Design review of the part built by this model. Coordinates are the model's own, in mm. Round coordinates to 2 decimals unless told otherwise and drop trailing zeros. Order: outer loops, then holes, each group sorted by start corner. A loop starts at its lowest first (then second) coordinate and runs counter-clockwise, first axis right, second up. Notation, with made-up numbers: (-11, -23) - (33, -23) arc R33 cw to (33, 5) - close; hole circle Ø4 at (-25.5, 47.5). An arc over 180 degrees is marked (long way). Use CSV: the item, a comma, the result in double quotes.
from build123d import *

# Parameters (mm, degrees)
SKETCH_1_W                = 188
SKETCH_1_H                = 150
EXTRUDE_1_DEPTH           = 2
SKETCH_13_W               = 188
SKETCH_13_H               = 12
CUT_EXTRUDE_8_DEPTH       = 11
SKETCH_5_R                = 1
EPP_DEPTH                 = 2
SKETCH_6_R                = 1
CUT_EXTRUDE_4_DEPTH       = 2
B_FAN_DEPTH               = 2
PCI_E_DEPTH               = 2
SKETCH_14_R               = 1
CUT_EXTRUDE_7447_DEPTH    = 5
IO_2_DEPTH                = 10
HOLE_WIZARD_1_AT_2_COUNT  = 2
HOLE_WIZARD_1_AT_2_PITCH  = 115.8
HOLE_WIZARD_1_AT_3_COUNT  = 2
HOLE_WIZARD_1_AT_3_PITCH  = 132.697701563
HOLE_WIZARD_1_AT_4_COUNT  = 2
HOLE_WIZARD_1_AT_4_PITCH  = 105.840068027
HOLE_WIZARD_1_AT_5_COUNT  = 2
HOLE_WIZARD_1_AT_5_PITCH  = 150.067318228
HOLE_WIZARD_1_AT_6_COUNT  = 2
HOLE_WIZARD_1_AT_6_PITCH  = 108.209056922
HOLE_WIZARD_1_AT_7_COUNT  = 2
HOLE_WIZARD_1_AT_7_PITCH  = 19.776754031
HOLE_WIZARD_1_AT_8_COUNT  = 2
HOLE_WIZARD_1_AT_8_PITCH  = 114.604799201
HOLE_WIZARD_1_AT_9_COUNT  = 2
HOLE_WIZARD_1_AT_9_PITCH  = 163.276483304
HOLE_WIZARD_1_AT_10_COUNT = 2
HOLE_WIZARD_1_AT_10_PITCH = 128.548084389
CUT_EXTRUDE_14_DEPTH      = 10
FILLET_2_R                = 1


with BuildPart() as part:
    # 草图1 → 凸台-拉伸1 (new body)
    with BuildSketch(Plane(origin=(0, 0, 0), x_dir=(0, 0, -1), z_dir=(1, 0, 0))):
        with Locations((-63.845257573, 68.271545487)):
            Rectangle(SKETCH_1_W, SKETCH_1_H)
    extrude(amount=EXTRUDE_1_DEPTH)

    # 草图13 → 切除-拉伸8 (cut)
    with BuildSketch(Plane(origin=(2, 0, 0), x_dir=(0, 0, -1), z_dir=(1, 0, 0))):
        with Locations((-63.845257573, 137.271545487)):
            Rectangle(SKETCH_13_W, SKETCH_13_H)
    extrude(amount=-CUT_EXTRUDE_8_DEPTH, mode=Mode.SUBTRACT)

    # 草图5 → EPP (cut)
    with BuildSketch(Plane.ZY):
        with Locations((40.345257573, 125.671545487)):
            Circle(SKETCH_5_R)
        with Locations((-24.454742427, 9.871545487)):
            Circle(SKETCH_5_R)
        with Locations((40.345257573, 9.871545487)):
            Circle(SKETCH_5_R)
    extrude(amount=-EPP_DEPTH, mode=Mode.SUBTRACT)

    # 草图6 → 切除-拉伸4 (cut)
    with BuildSketch(Plane.ZY):
        with Locations((57.745257573, 116.271545487)):
            Circle(SKETCH_6_R)
        with Locations((148.145257573, 116.271545487)):
            Circle(SKETCH_6_R)
        with Locations((57.745257573, 21.271545487)):
            Circle(SKETCH_6_R)
        with Locations((148.145257573, 21.271545487)):
            Circle(SKETCH_6_R)
    extrude(amount=-CUT_EXTRUDE_4_DEPTH, mode=Mode.SUBTRACT)

    # 草图3 → B-FAN (cut)
    with BuildSketch(Plane.ZY):
        Polygon((-30.154742427, -6.728454513), (46.845257573, -6.728454513), (46.845257573, 4.271545487), (46.845257573, 5.271545487), (36.845257573, 5.271545487), (36.845257573, 4.271545487), (-20.154742427, 4.271545487), (-20.154742427, 5.271545487), (-30.154742427, 5.271545487), (-30.154742427, 4.271545487), align=None)
    extrude(amount=-B_FAN_DEPTH, mode=Mode.SUBTRACT)

    # 草图10 → PCI-E (cut)
    with BuildSketch(Plane.ZY):
        Polygon((46.845257573, 5.271545487), (46.845257573, -6.728454513), (157.845257573, -6.728454513), (157.845257573, 5.271545487), (151.845257573, 5.271545487), (151.845257573, 17.271545487), (46.845257573, 17.271545487), align=None)
    extrude(amount=-PCI_E_DEPTH, mode=Mode.SUBTRACT)

    # 草图14 → Cut-Extrude 7447 (cut)
    with BuildSketch(Plane.ZY):
        with Locations((154.845257573, 120.771545487)):
            Circle(SKETCH_14_R)
        with Locations((154.845257573, 9.271545487)):
            Circle(SKETCH_14_R)
        with Locations((-27.154742427, 16.271545487)):
            Circle(SKETCH_14_R)
        with Locations((-27.154742427, 120.271545487)):
            Circle(SKETCH_14_R)
    extrude(amount=-CUT_EXTRUDE_7447_DEPTH, mode=Mode.SUBTRACT)

    # 草图15 → IO 2 (cut)
    with BuildSketch(Plane.ZY):
        Polygon((157.845257573, 118.271545487), (156.345257573, 118.271545487), (151.145257573, 118.271545487), (151.145257573, 113.771545487), (156.345257573, 113.771545487), (156.345257573, 12.271545487), (157.845257573, 12.271545487), align=None)
    extrude(amount=-IO_2_DEPTH, mode=Mode.SUBTRACT)

    # 草图17 → 打孔尺寸(%根据)内六角花形沉头螺钉的类型1 (revolve, cut)
    with BuildSketch(Plane(origin=(2, 125.671545487, 40.345257573), x_dir=(0, 0, -1), z_dir=(0, 1, 0))):
        Polygon((0, 0), (0, 2), (1.1, 2), (1.1, 1.1), (2.2, 0), align=None)
    hole_wizard_1 = revolve(axis=Axis((8.35, 125.671545487, 40.345257573), (-1, 0, 0)), mode=Mode.SUBTRACT)

    # 打孔尺寸(%根据)内六角花形沉头螺钉的类型1 at 2: 打孔尺寸(%根据)内六角花形沉头螺钉的类型1 ×2
    with Locations(*[(0, -i * HOLE_WIZARD_1_AT_2_PITCH, 0) for i in range(1, HOLE_WIZARD_1_AT_2_COUNT)]):
        add(hole_wizard_1, mode=Mode.SUBTRACT)

    # 打孔尺寸(%根据)内六角花形沉头螺钉的类型1 at 3: 打孔尺寸(%根据)内六角花形沉头螺钉的类型1 ×2
    with Locations(*[Vector(0, -0.8726601790111727, -0.4883279758197234) * (i * HOLE_WIZARD_1_AT_3_PITCH) for i in range(1, HOLE_WIZARD_1_AT_3_COUNT)]):
        add(hole_wizard_1, mode=Mode.SUBTRACT)

    # 打孔尺寸(%根据)内六角花形沉头螺钉的类型1 at 4: 打孔尺寸(%根据)内六角花形沉头螺钉的类型1 ×2
    with Locations(*[Vector(0, -0.9863939238321437, 0.16439898730535765) * (i * HOLE_WIZARD_1_AT_4_PITCH) for i in range(1, HOLE_WIZARD_1_AT_4_COUNT)]):
        add(hole_wizard_1, mode=Mode.SUBTRACT)

    # 打孔尺寸(%根据)内六角花形沉头螺钉的类型1 at 5: 打孔尺寸(%根据)内六角花形沉头螺钉的类型1 ×2
    with Locations(*[Vector(0, -0.6956877835433596, 0.7183442822411324) * (i * HOLE_WIZARD_1_AT_5_PITCH) for i in range(1, HOLE_WIZARD_1_AT_5_COUNT)]):
        add(hole_wizard_1, mode=Mode.SUBTRACT)

    # 打孔尺寸(%根据)内六角花形沉头螺钉的类型1 at 6: 打孔尺寸(%根据)内六角花形沉头螺钉的类型1 ×2
    with Locations(*[Vector(0, -0.0868688838749896, 0.9962197533748834) * (i * HOLE_WIZARD_1_AT_6_PITCH) for i in range(1, HOLE_WIZARD_1_AT_6_COUNT)]):
        add(hole_wizard_1, mode=Mode.SUBTRACT)

    # 打孔尺寸(%根据)内六角花形沉头螺钉的类型1 at 7: 打孔尺寸(%根据)内六角花形沉头螺钉的类型1 ×2
    with Locations(*[Vector(0, -0.47530550186838766, 0.8798208226074444) * (i * HOLE_WIZARD_1_AT_7_PITCH) for i in range(1, HOLE_WIZARD_1_AT_7_COUNT)]):
        add(hole_wizard_1, mode=Mode.SUBTRACT)

    # 打孔尺寸(%根据)内六角花形沉头螺钉的类型1 at 8: 打孔尺寸(%根据)内六角花形沉头螺钉的类型1 ×2
    with Locations(*[Vector(0, -0.04275562658931698, 0.9990855600973096) * (i * HOLE_WIZARD_1_AT_8_PITCH) for i in range(1, HOLE_WIZARD_1_AT_8_COUNT)]):
        add(hole_wizard_1, mode=Mode.SUBTRACT)

    # 打孔尺寸(%根据)内六角花形沉头螺钉的类型1 at 9: 打孔尺寸(%根据)内六角花形沉头螺钉的类型1 ×2
    with Locations(*[Vector(0, -0.7129011946168821, 0.7012644912683248) * (i * HOLE_WIZARD_1_AT_9_PITCH) for i in range(1, HOLE_WIZARD_1_AT_9_COUNT)]):
        add(hole_wizard_1, mode=Mode.SUBTRACT)

    # 打孔尺寸(%根据)内六角花形沉头螺钉的类型1 at 10: 打孔尺寸(%根据)内六角花形沉头螺钉的类型1 ×2
    with Locations(*[Vector(0, -0.8510434093223341, -0.5250953393899228) * (i * HOLE_WIZARD_1_AT_10_PITCH) for i in range(1, HOLE_WIZARD_1_AT_10_COUNT)]):
        add(hole_wizard_1, mode=Mode.SUBTRACT)

    # 草图23 → 切除-拉伸14 (cut)
    with BuildSketch(Plane.ZY):
        with BuildLine():
            Line((83.595257573, 133.521545487), (83.595257573, 129.021545487))
            ThreePointArc((83.595257573, 129.021545487), (81.345257573, 126.771545487), (79.095257573, 129.021545487))
            Line((79.095257573, 129.021545487), (79.095257573, 133.521545487))
            ThreePointArc((79.095257573, 133.521545487), (81.345257573, 135.771545487), (83.595257573, 133.521545487))
        make_face()
    extrude(amount=-CUT_EXTRUDE_14_DEPTH, mode=Mode.SUBTRACT)

    # 圆角2
    fillet_2_edges = [part.edges().sort_by_distance(p)[0] for p in [
        (1, 113.771545487, 151.145257573),
        (1, 118.271545487, 151.145257573),
        (1, 12.271545487, 156.345257573),
        (1, 17.271545487, 151.845257573),
        (1, 17.271545487, 46.845257573),
        (1, 5.271545487, 36.845257573),
        (1, 5.271545487, -20.154742427),
    ]]
    fillet(fillet_2_edges, radius=FILLET_2_R - 0.0001)  # a hair under: the kernel refuses the full size


solid = part.part
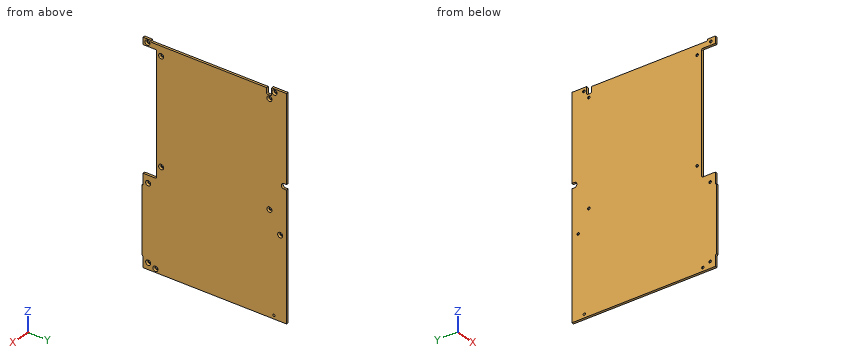
1) Insertion check: pin 1 Ø1 at (x, y) = (1, 116.5) entering from +Z; pin 2 Ø0.6 at (x, z) = (1, 156) entering from -Y; pin 3 Ø1 at (x, y) = (1.5, 43.5) entering from +Z; pin 4 Ø1.8 at (y, z) = (116.27, 57.75) entering from -X. Each pin has a flat end and moves straight along its axis. Give the tip position at first contact, or say it passes through.
Data:
pin 1,"stops at z = 151.15"
pin 2,"stops at y = 5.27"
pin 3,"stops at z = 156.35"
pin 4,"passes through"
2) We need section A-A (z = 136). Give the boundary of the cut face in (x, y), then the cut area to 3 significant figures.
Data:
outline,"(0, 17.27) - (2, 17.27) - (2, 131.27) - (0, 131.27) - close"
area,"228 mm2"
3) We need section B-B (x = 0.35). Give the number of separate pieces and of enclosed holes in the cut face, then the cut area to 3 significant figures.
Data:
separate pieces,"1"
enclosed holes,"11"
area,"22,200 mm2"
4) To check wall thickness, follow L1, parallel to Z at x = 0.5, y = 21; L2, parallel to Y at x = 1.95, z = 150; L3, parallel to Z at x = 1.8, y = 108. State the ranges of each line that lie inside material, in increasing order. Write a range as from..to.
Data:
L1,"z = -30.15..56.68, 58.81..147.08, 149.21..156.35"
L2,"y = 17.27..20.18, 22.36..115.18, 117.36..131.27"
L3,"z = -30.15..156.35"
